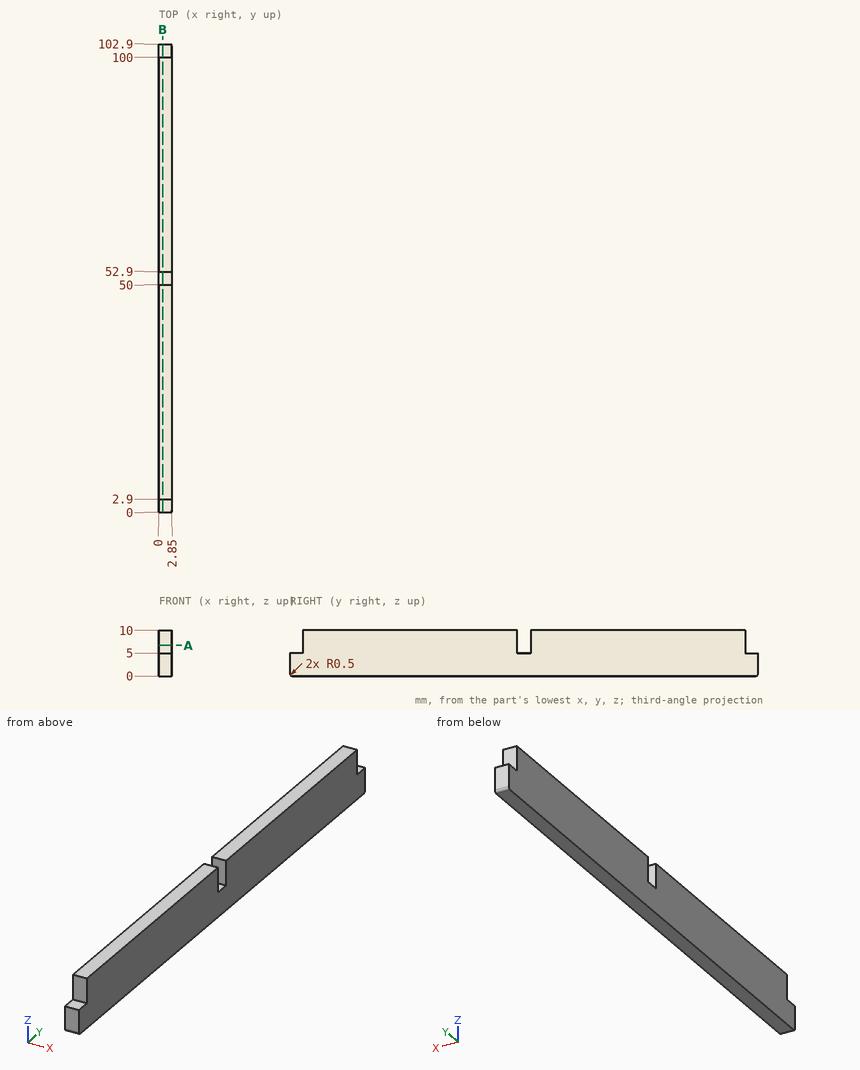
Check sheet for the drawn part. Datum: minimum x, y, z corner. Units: mm. Give positions to 0.01 mm unless a question says otherwise; leave off trailing zeros. Order: outer loops, then holes, each group sorted by start corner. A loop starts at its lowest first (then second) coordinate and runs counter-clockwise, first axis right, second up.
1. Sectioned sample at B-B (x = 0.85). Record the boundary of the cut face in (y, z), then the cut area to 3 significant figures.
Completed:
outline: (0, 0.5) arc R0.5 ccw to (0.5, 0) - (102.4, 0) arc R0.5 ccw to (102.9, 0.5) - (102.9, 5) - (100, 5) - (100, 10) - (52.9, 10) - (52.9, 5) - (50, 5) - (50, 10) - (2.9, 10) - (2.9, 5) - (0, 5) - close
area: 985 mm2
2. Scan lines: line 1 (Y direction, x = 1.2, z = 7.5); line 2 (Z direction, x = 2.35, y = 52.5). Record each from-to range of solid material in increasing order.
Completed:
line 1: y = 2.9 to 50, 52.9 to 100
line 2: z = 0 to 5
3. Sectioned sample at A-A (z = 6.75). Record the boundary of the cut face in (x, y).
Completed:
outline: (0, 2.9) - (2.85, 2.9) - (2.85, 50) - (0, 50) - close; (0, 52.9) - (2.85, 52.9) - (2.85, 100) - (0, 100) - close
4. Depth check by flat-ended pin: pin 1 (1.4 mm diameter, centred on x = 1.5, y = 101, fed in from +Z); pin 2 (1.4 mm diameter, centred on x = 2, z = 8, fed in from +Y). Enter the tip coordinate at first touch or a pass-through.
Completed:
pin 1: stops at z = 5
pin 2: stops at y = 100
